```python
from build123d import *

# Parameters (mm, degrees)
SKETCH1_W           = 125
SKETCH1_H           = 125
BOSS_EXTRUDE1_DEPTH = 200
SHELL1_T            = -10
SKETCH2_W           = 135
SKETCH2_H           = 135
SKETCH2_W_2         = 125
SKETCH2_H_2         = 125
SKETCH2_W_3         = 105
SKETCH2_H_3         = 105
BOSS_EXTRUDE2_DEPTH = 5
SKETCH3_W           = 135
SKETCH3_H           = 135
SKETCH3_W_2         = 125
SKETCH3_H_2         = 125
SKETCH3_W_3         = 105
SKETCH3_H_3         = 105
BOSS_EXTRUDE3_DEPTH = 5


with BuildPart() as part:
    # Sketch1 → Boss-Extrude1 (new body)
    with BuildSketch(Plane.XY):
        Rectangle(SKETCH1_W, SKETCH1_H)
    extrude(amount=BOSS_EXTRUDE1_DEPTH)

    # Shell1
    shell1_openings = [part.faces().sort_by_distance(p)[0] for p in [
        (0, 0, 200),
        (0, 0, 0),
    ]]
    offset(amount=SHELL1_T, openings=shell1_openings, kind=Kind.INTERSECTION)

    # Sketch2 → Boss-Extrude2 (add)
    # profile 1 of 2: a face of its own
    with BuildSketch(Plane.XY.offset(200)):
        Rectangle(SKETCH2_W, SKETCH2_H)
        Rectangle(SKETCH2_W_2, SKETCH2_H_2, mode=Mode.SUBTRACT)
    # profile 2 of 2: a face of its own
    with BuildSketch(Plane.XY.offset(200)):
        Rectangle(SKETCH2_W_2, SKETCH2_H_2)
        Rectangle(SKETCH2_W_3, SKETCH2_H_3, mode=Mode.SUBTRACT)
    extrude(amount=-BOSS_EXTRUDE2_DEPTH)

    # Sketch3 → Boss-Extrude3 (add)
    # profile 1 of 2: a face of its own
    with BuildSketch(Plane(origin=(0, 0, 0), x_dir=(-1, 0, 0), z_dir=(0, 0, -1))):
        Rectangle(SKETCH3_W, SKETCH3_H)
        Rectangle(SKETCH3_W_2, SKETCH3_H_2, mode=Mode.SUBTRACT)
    # profile 2 of 2: a face of its own
    with BuildSketch(Plane(origin=(0, 0, 0), x_dir=(-1, 0, 0), z_dir=(0, 0, -1))):
        Rectangle(SKETCH3_W_2, SKETCH3_H_2)
        Rectangle(SKETCH3_W_3, SKETCH3_H_3, mode=Mode.SUBTRACT)
    extrude(amount=-BOSS_EXTRUDE3_DEPTH)


solid = part.part
```
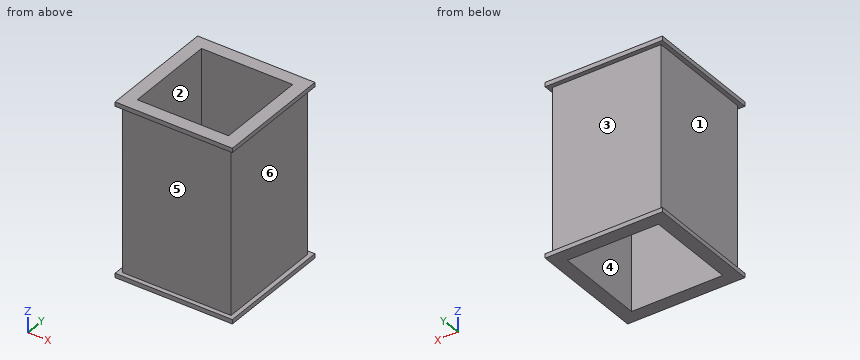
Can you work these out from the model? Positions are in its coordinate system, mm. Face numbers are marked on the shaded views. A direction names the side the tool comes from. Coordinates: 2 decimals unless noted, no trailing zeros. Loops run counter-clockwise (first coordinate to the right, second up) from the corner with the lowest first, then second, coordinate; pieces in that order, holes last. Notation, with made-up numbers: (15.25, -22.75) - (66.25, -22.75) arc R31 ccw to (66.25, 3.25) - close; hole circle Ø2 at (18.25, -16.5). An arc over 180 degrees is marked (long way). Answer as CSV lines item,"result". Start each with the question number.
1) Thinking about a two-plate mould opening in X: for the marked faces 1, 2 and 3, which applies, pulls with the +X half, pulls with the -X half, needs draft (parallel to the pull), parting line crosses it, or undercut?
2) Suppose I cut it at A-A (y = 36). Please give me the cut outline in (x, z), plus the area to 3 significant figures.
3) I need wall thicknesses on line 1 (Y direction, x = -39, z = 66.5); line 2 (Y direction, x = -59.5, z = 184.5). Which ranges of each line are inside material? Lowest first, please. Write a range as from..to.
4) For pin 1 (5 mm diameter, centred on y = 49.5, z = 146.5, fed in from +X); pin 2 (4 mm diameter, centred on y = 8.5, z = 97, fed in from -X); pin 3 (10 mm diameter, centred on x = -52.5, z = 86, fed in from -Y), each with a flat end and sliding along its axis, tell me the tip position at first contact or that it passes through.
5) Suppose I cut it at C-C (z = 13). Please give me the cut outline in (x, y), plus the area to 3 significant figures.
6) Which directions (+Z, -Z, +X, -X, +Y, -Y) give clear straight access to the entire face, cutting with the end or side of a thin tool? Please do the marked faces 4, 5 and 6.
Check result:
1,face 1,"pulls with the -X half"
1,face 2,"undercut"
1,face 3,"needs draft"
2,outline,"(-67.5, 0) - (-52.5, 0) - (-52.5, 200) - (-67.5, 200) - (-67.5, 195) - (-62.5, 195) - (-62.5, 5) - (-67.5, 5) - close; (52.5, 0) - (67.5, 0) - (67.5, 5) - (62.5, 5) - (62.5, 195) - (67.5, 195) - (67.5, 200) - (52.5, 200) - close"
2,area,"4,100 mm²"
3,line 1,"y = -62.5..-52.5, 52.5..62.5"
3,line 2,"y = -62.5..62.5"
4,pin 1,"stops at x = 62.5"
4,pin 2,"stops at x = -62.5"
4,pin 3,"stops at y = -62.5"
5,outline,"(-62.5, -62.5) - (62.5, -62.5) - (62.5, 62.5) - (-62.5, 62.5) - close; hole (-52.5, -52.5) - (52.5, -52.5) - (52.5, 52.5) - (-52.5, 52.5) - close"
5,area,"4,600 mm²"
6,face 4,"+Z, -Z"
6,face 5,"+X, -X, -Y"
6,face 6,"+X, +Y, -Y"
